Model file for the job. Use its own axes, mm. Face numbers are marked on the shaded views. A direction names the side the tool comes from. Give positions to 0.01 mm unless a question says otherwise; leave off trailing zeros. Order: outer loops, then holes, each group sorted by start corner. A loop starts at its lowest first (then second) coordinate and runs counter-clockwise, first axis right, second up. Notation, with made-up numbers: M 32.25,-35 L 82.25,-35 A17 ccw 82.25,-10 Z; hole C 83.25,83.5 d7. An arc over 180 degrees is marked long. Return JSON: item names as keys, results as strings. Group by question number.
1. Slice it at C-C on z = 33.5. List the corners of the cut face in (x, y).
2. Two-plate mould, pull along Z, no slides. Class the marked faces 5, 6, 7 and 8: released by +Z, released by -Z, zero draft, split by the parting line, or undercut.
3. Slice it at B-B on x = -59.66. List the corners of the cut face in (y, z), then the cut area to 3 significant figures.
4. Pin check, flat tips, straight feed: pin 1 (5.5 mm diameter, centred on x = -59.66, z = 54.86, fed in from -Y); pin 2 (8 mm diameter, centred on x = -45.5, z = 58.5, fed in from +Y); pin 3 (0.8 mm diameter, centred on y = -1.5, z = 61.5, fed in from -X). Stop position of each tip, or through.
5. Slice it at A-A on z = 6.16. List the corners of the cut face in (x, y).
6. 3-axis set-ups, long thin cutter, end or side, ignore diameter. For the marked faces 1, 2, 3 and 4: which of +Z, -Z, +X, -X, +Y, -Y reach the whole face in a straight line?
7. Wall check: probe 1 along X at (y, z) = (-11.25, 45); probe 2 along X at (y, z) = (-7, 6.16); probe 3 along X at (y, z) = (-1.75, 30). Give the ranges that are in metal, low to high. Write a range as [from, to].
8. Slice it at D-D on x = -15. List the corners of the cut face in (y, z).
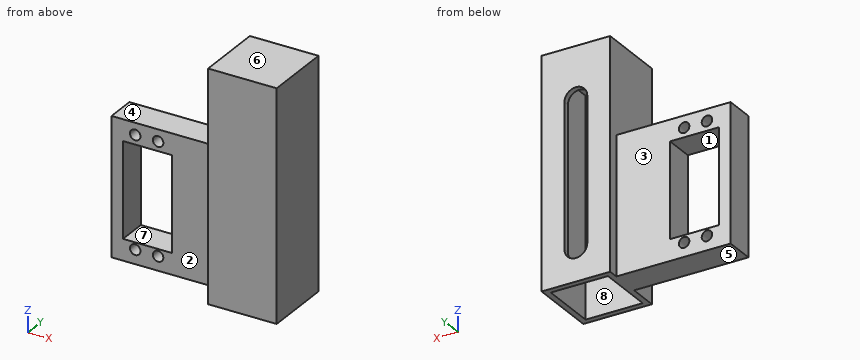
from build123d import *

# Parameters (mm, degrees)
ESQUISSE1_W             = 30
ESQUISSE1_H             = 30
BOSS_EXTRU_1_DEPTH      = 100
ESQUISSE2_W             = 25
ESQUISSE2_H             = 25
ENL_V_MAT_EXTRU_1_DEPTH = 95
ENL_V_MAT_EXTRU_2_DEPTH = 2.5
ESQUISSE4_W             = 60
ESQUISSE4_H             = 25.6
BOSS_EXTRU_2_DEPTH      = 50
ESQUISSE5_W             = 21.5
ESQUISSE5_H             = 41.5
ENL_V_MAT_EXTRU_3_DEPTH = 132.52946438
ESQUISSE6_R             = 2.3
ENL_V_MAT_EXTRU_4_DEPTH = 132.52946438
ESQUISSE9_W             = 50
ESQUISSE9_H             = 12.8
ENL_V_MAT_EXTRU_6_DEPTH = 132.52946438


with BuildPart() as part:
    # Esquisse1 → Boss.-Extru.1 (new body)
    with BuildSketch(Plane.XY):
        with Locations((-15, -15)):
            Rectangle(ESQUISSE1_W, ESQUISSE1_H)
    extrude(amount=BOSS_EXTRU_1_DEPTH)

    # Esquisse2 → Enlèv. mat.-Extru.1 (cut)
    with BuildSketch(Plane(origin=(0, 0, 0), x_dir=(-1, 0, 0), z_dir=(0, 0, -1))):
        with Locations((15, -15)):
            Rectangle(ESQUISSE2_W, ESQUISSE2_H)
    extrude(amount=-ENL_V_MAT_EXTRU_1_DEPTH, mode=Mode.SUBTRACT)

    # Esquisse3 → Enlèv. mat.-Extru.2 (cut)
    with BuildSketch(Plane(origin=(0, 0, 0), x_dir=(1, 0, 0), z_dir=(0, 1, 0))):
        with BuildLine():
            Line((-10, -15), (-10, -77.5))
            ThreePointArc((-10, -77.5), (-15, -82.5), (-20, -77.5))
            Line((-20, -77.5), (-20, -15))
            ThreePointArc((-20, -15), (-15, -10), (-10, -15))
        make_face()
    extrude(amount=-ENL_V_MAT_EXTRU_2_DEPTH, mode=Mode.SUBTRACT)

    # Esquisse4 → Boss.-Extru.2 (add)
    with BuildSketch(Plane.ZY.offset(30)):
        with Locations((30, -17.2)):
            Rectangle(ESQUISSE4_W, ESQUISSE4_H)
    extrude(amount=BOSS_EXTRU_2_DEPTH)

    # Esquisse5 → Enlèv. mat.-Extru.3 (cut, through all)
    with BuildSketch(Plane(origin=(0, 0, 0), x_dir=(1, 0, 0), z_dir=(0, 1, 0))):
        with Locations((-64.25, -30)):
            Rectangle(ESQUISSE5_W, ESQUISSE5_H)
    extrude(amount=-ENL_V_MAT_EXTRU_3_DEPTH, mode=Mode.SUBTRACT)

    # Esquisse6 → Enlèv. mat.-Extru.4 (cut, through all)
    with BuildSketch(Plane(origin=(0, 0, 0), x_dir=(1, 0, 0), z_dir=(0, 1, 0))):
        with Locations(Location((-69.66, -54.86, 0), (0, 0, 270))):
            Circle(ESQUISSE6_R)
        with Locations(Location((-59.66, -54.86, 0), (0, 0, 270))):
            Circle(ESQUISSE6_R)
        with Locations(Location((-69.66, -6.16, 0), (0, 0, 270))):
            Circle(ESQUISSE6_R)
        with Locations(Location((-59.66, -6.16, 0), (0, 0, 270))):
            Circle(ESQUISSE6_R)
    extrude(amount=-ENL_V_MAT_EXTRU_4_DEPTH, mode=Mode.SUBTRACT)

    # Esquisse9 → Enlèv. mat.-Extru.6 (cut, through all)
    with BuildSketch(Plane(origin=(0, 0, 0), x_dir=(-1, 0, 0), z_dir=(0, 0, -1))):
        with Locations((55, -23.6)):
            Rectangle(ESQUISSE9_W, ESQUISSE9_H)
    extrude(amount=-ENL_V_MAT_EXTRU_6_DEPTH, mode=Mode.SUBTRACT)


solid = part.part
Result:
{
 "1": {"outline": "M -80,-17.2 L -75,-17.2 L -75,-4.4 L -80,-4.4 Z; M -53.5,-17.2 L -30,-17.2 L -30,-30 L 0,-30 L 0,0 L -10,0 L -10,-2.5 L -2.5,-2.5 L -2.5,-27.5 L -27.5,-27.5 L -27.5,-2.5 L -20,-2.5 L -20,0 L -30,0 L -30,-4.4 L -53.5,-4.4 Z"},
 "2": {"face 5": "released by -Z", "face 6": "released by +Z", "face 7": "undercut", "face 8": "zero draft"},
 "3": {"outline": "M -17.2,0 L -4.4,0 L -4.4,3.86 L -17.2,3.86 Z; M -17.2,8.46 L -4.4,8.46 L -4.4,9.25 L -17.2,9.25 Z; M -17.2,50.75 L -4.4,50.75 L -4.4,52.56 L -17.2,52.56 Z; M -17.2,57.16 L -4.4,57.16 L -4.4,60 L -17.2,60 Z", "area": "119 mm2"},
 "4": {"pin 1": "stops at y = -17.2", "pin 2": "stops at y = -4.4", "pin 3": "stops at x = -30"},
 "5": {"outline": "M -80,-17.2 L -71.96,-17.2 L -71.96,-4.4 L -80,-4.4 Z; M -67.36,-17.2 L -61.96,-17.2 L -61.96,-4.4 L -67.36,-4.4 Z; M -57.36,-17.2 L -30,-17.2 L -30,-30 L 0,-30 L 0,0 L -30,0 L -30,-4.4 L -57.36,-4.4 Z; hole M -27.5,-27.5 L -2.5,-27.5 L -2.5,-2.5 L -27.5,-2.5 Z"},
 "6": {"face 1": "+Y, -Y", "face 2": "+Z, -Z, -X, -Y", "face 3": "+Z, -Z, -X, +Y", "face 4": "+Z, -X, +Y, -Y"},
 "7": {"probe 1": "x = [-80, -75], [-53.5, -27.5], [-2.5, 0]", "probe 2": "x = [-80, -71.96], [-67.36, -61.96], [-57.36, -27.5], [-2.5, 0]", "probe 3": "x = [-30, -20], [-10, 0]"},
 "8": {"outline": "M -30,0 L -27.5,0 L -27.5,95 L -2.5,95 L -2.5,82.5 L 0,82.5 L 0,100 L -30,100 Z; M -2.5,0 L 0,0 L 0,10 L -2.5,10 Z"}
}
